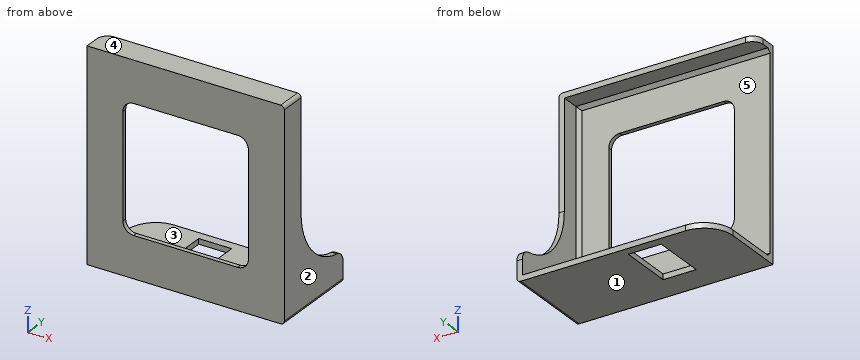
```python
from build123d import *

# Parameters (mm, degrees)
ESBO_O1_W             = 55
ESBO_O1_H             = 58
BASE_DEPTH            = 1.2
ESBO_O2_W             = 55
ESBO_O2_H             = 58
ESBO_O2_W_2           = 52
ESBO_O2_H_2           = 55
PAREDES_DEPTH         = 24
ESBO_O3_W             = 4.971937724
ESBO_O3_H             = 55
CORTE_EXTRUS_O1_DEPTH = 24
ESBO_O4_W             = 9.2
ESBO_O4_H             = 15
ENCAIXE_CHAVE_DEPTH   = 17
ESBO_O5_W             = 1.5
ESBO_O5_H             = 18
CORTE_EXTRUS_O3_DEPTH = 68.089790579
ESBO_O6_W             = 30
ESBO_O6_H             = 18
CORTE_EXTRUS_O4_DEPTH = 17
FILETE1_R             = 8
FILETE2_R             = 3
FILETE3_R             = 3
FILETE4_R             = 1
FILETE5_R             = 1
CHANFRO1_SIZE         = 1
CORTE_EXTRUS_O5_DEPTH = 17


with BuildPart() as part:
    # Esboço1 → Base (new body)
    with BuildSketch(Plane(origin=(0, 0, 0), x_dir=(1, 0, 0), z_dir=(0, 1, 0))):
        Rectangle(ESBO_O1_W, ESBO_O1_H)
    extrude(amount=BASE_DEPTH)

    # Esboço2 → Paredes (add)
    with BuildSketch(Plane(origin=(0, 1.2, 0), x_dir=(1, 0, 0), z_dir=(0, 1, 0))):
        Rectangle(ESBO_O2_W, ESBO_O2_H)
        Rectangle(ESBO_O2_W_2, ESBO_O2_H_2, mode=Mode.SUBTRACT)
    extrude(amount=PAREDES_DEPTH)

    # Esboço3 → Corte-extrusão1 (cut)
    with BuildSketch(Plane(origin=(0, 25.2, 0), x_dir=(1, 0, 0), z_dir=(0, 1, 0))):
        with Locations((-27.5, 0)):
            Rectangle(ESBO_O3_W, ESBO_O3_H)
    extrude(amount=-CORTE_EXTRUS_O1_DEPTH, mode=Mode.SUBTRACT)

    # Esboço4 → Encaixe chave (cut)
    with BuildSketch(Plane(origin=(0, 0, -29), x_dir=(-1, 0, 0), z_dir=(0, 0, -1))):
        with Locations((6.5, 15.2)):
            Rectangle(ESBO_O4_W, ESBO_O4_H)
    extrude(amount=-ENCAIXE_CHAVE_DEPTH, mode=Mode.SUBTRACT)

    # Esboço5 → Corte-extrusão3 (cut, through all)
    with BuildSketch(Plane.ZY.offset(27.5)):
        with Locations((28.25, 16.2)):
            Rectangle(ESBO_O5_W, ESBO_O5_H)
    extrude(amount=-CORTE_EXTRUS_O3_DEPTH, mode=Mode.SUBTRACT)

    # Esboço6 → Corte-extrusão4 (cut)
    with BuildSketch(Plane(origin=(27.5, 0, 0), x_dir=(0, 0, -1), z_dir=(1, 0, 0))):
        with BuildLine():
            Line((20.5, 25.2), (2.5, 25.2))
            Line((2.5, 25.2), (2.5, 7.2))
            ThreePointArc((2.5, 7.2), (15.227922061, 12.472077939), (20.5, 25.2))
        make_face()
        with Locations((-12.5, 16.2)):
            Rectangle(ESBO_O6_W, ESBO_O6_H)
    extrude(amount=-CORTE_EXTRUS_O4_DEPTH, mode=Mode.SUBTRACT)

    # Filete1
    filete1_edges = [part.edges().sort_by_distance(p)[0] for p in [
        (-27.5, 25.2, -28.25),
    ]]
    fillet(filete1_edges, radius=FILETE1_R)

    # Filete2
    filete2_edges = [part.edges().sort_by_distance(p)[0] for p in [
        (-27.5, 7.2, 28.25),
    ]]
    fillet(filete2_edges, radius=FILETE2_R)

    # Filete3
    filete3_edges = [part.edges().sort_by_distance(p)[0] for p in [
        (26.75, 25.2, -20.5),
    ]]
    fillet(filete3_edges, radius=FILETE3_R)

    # Filete4
    filete4_edges = [part.edges().sort_by_distance(p)[0] for p in [
        (27.5, 3.6, 29),
    ]]
    fillet(filete4_edges, radius=FILETE4_R)

    # Filete5
    filete5_edges = [part.edges().sort_by_distance(p)[0] for p in [
        (27.5, 12.6, -29),
    ]]
    fillet(filete5_edges, radius=FILETE5_R)

    # Chanfro1
    chanfro1_edges = [part.edges().sort_by_distance(p)[0] for p in [
        (26, 1.2, 0),
        (-0.75, 1.2, -27.5),
        (-0.75, 1.2, 27.5),
    ]]
    chamfer(chanfro1_edges, length=CHANFRO1_SIZE)

    # Esboço7 → Corte-extrusão5 (cut)
    with BuildSketch(Plane(origin=(0, 1.2, 0), x_dir=(1, 0, 0), z_dir=(0, 1, 0))):
        with BuildLine():
            Line((-14.5, -17.5), (14.5, -17.5))
            ThreePointArc((14.5, -17.5), (16.621320344, -16.621320344), (17.5, -14.5))
            Line((17.5, -14.5), (17.5, 14.5))
            ThreePointArc((17.5, 14.5), (16.621320344, 16.621320344), (14.5, 17.5))
            Line((14.5, 17.5), (-14.5, 17.5))
            ThreePointArc((-14.5, 17.5), (-16.621320344, 16.621320344), (-17.5, 14.5))
            Line((-17.5, 14.5), (-17.5, -14.5))
            ThreePointArc((-17.5, -14.5), (-16.621320344, -16.621320344), (-14.5, -17.5))
        make_face()
    extrude(amount=-CORTE_EXTRUS_O5_DEPTH, mode=Mode.SUBTRACT)


solid = part.part
```
Check sheet for the modelled part. Datum: model origin and axes. Units: mm. Face numbers are marked on the shaded views. A direction names the side the tool comes from. Coordinates: 2 decimals unless noted, no trailing zeros. Loops run counter-clockwise (first coordinate to the right, second up) from the corner with the lowest first, then second, coordinate; pieces in that order, holes last.
1) Material ranges on probe 1 along Z at (x, y) = (-4.5, 7.5); probe 2 along Z at (x, y) = (-2.5, 5.25); probe 3 along Y at (x, z) = (21.5, -24.5), recorded low to high.
2) Gauge pin test, flat ends, axial feed: pin 1 (8 mm diameter, centred on x = -14, z = -5, fed in from +Y); pin 2 (0.8 mm diameter, centred on y = 12.5, z = -28.5, fed in from +X) (3 decimals). Record the tip position at first contact, or that the pin passes through.
3) Sectioned sample at D-D (y = 20.25). Record the boundary of the cut face in (x, z), and give its area (3 significant figures).
4) Sectioned sample at A-A (x = -5). Record the boundary of the cut face in (y, z), and give its area (3 significant figures).
5) Sectioned sample at C-C (x = -12). Record the boundary of the cut face in (y, z).
6) Release check for a two-part mould opening along Z. For the marked faces 1, 2 and 3 record: released by +Z, released by -Z, zero draft, split by the parting line, or undercut.
7) Sectioned sample at B-B (z = 5.5). Record the boundary of the cut face in (x, y).
8) Access from +Z, -Z, +X, -X, +Y, -Y to the whole of each face (thin tool, end or side, straight path). Record for the marked faces 4 and 5.
Check sheet entries:
1. probe 1: z = -29 to -27.5
1. probe 2: z = -29 to -27.5, 27.5 to 29
1. probe 3: y = 0 to 1.2
2. pin 1: stops at y = 1.2
2. pin 2: stops at x = 27.495
3. outline: (-26.9, -29) - (-11.1, -29) - (-11.1, -27.5) - (-26.9, -27.5) - close; (-1.9, -29) - (26.5, -29) arc R1 ccw to (27.5, -28) - (27.5, -19.81) - (26, -19.81) - (26, -27.5) - (-1.9, -27.5) - close
3. area: 79.1 mm2
4. outline: (0, -29) - (7.7, -29) - (7.7, -27.5) - (2.2, -27.5) - (1.2, -26.5) - (1.2, -17.5) - (0, -17.5) - close; (0, 17.5) - (1.2, 17.5) - (1.2, 26.5) - (2.2, 27.5) - (7.2, 27.5) - (7.2, 29) - (0, 29) - close; (22.7, -29) - (25.2, -29) - (25.2, -27.5) - (22.7, -27.5) - close
4. area: 51.1 mm2
5. outline: (0, -29) - (25.2, -29) - (25.2, -27.5) - (2.2, -27.5) - (1.2, -26.5) - (1.2, -17.5) - (0, -17.5) - close; (0, 17.5) - (1.2, 17.5) - (1.2, 26.5) - (2.2, 27.5) - (7.2, 27.5) - (7.2, 29) - (0, 29) - close
6. face 1: released by -Z
6. face 2: zero draft
6. face 3: undercut
7. outline: (-27.5, 0) - (-17.5, 0) - (-17.5, 1.2) - (-27.5, 1.2) - close; (17.5, 0) - (27.5, 0) - (27.5, 7.2) - (26, 7.2) - (26, 2.2) - (25, 1.2) - (17.5, 1.2) - close
8. face 4: +Z, +X, -X, +Y, -Y
8. face 5: -X, +Y
